Design review of the part built by this model. Coordinates are the model's own, in mm. Face numbers are marked on the shaded views. A direction names the side the tool comes from. Coordinates: 2 decimals unless noted, no trailing zeros. Write each loop counter-clockwise with the first axis right and the second up, starting at its lowest first coordinate (ties: lowest second). Pieces come first, ordered by that corner, then holes.
```python
from build123d import *

# Parameters (mm, degrees)
SKETCH1_W               = 54.356
SKETCH1_H               = 34.798
SKETCH1_R               = 1.250004527
SKETCH1_W_2             = 50.4000008
SKETCH1_H_2             = 5.2500022
BOSS_EXTRUDE1_DEPTH     = 1.999996
SKETCH2_W               = 54.356
SKETCH2_H               = 1.626997
BOSS_EXTRUDE2_DEPTH     = 4.1999916
SKETCH3_R               = 1.250004527
BOSS_EXTRUDE3_DEPTH     = 4.1999916
CUT_EXTRUDE1_DEPTH      = 33.88498208
CUT_EXTRUDE1_DEPTH_BACK = 33.88498208


with BuildPart() as part:
    # Sketch1 → Boss-Extrude1 (new body)
    with BuildSketch(Plane(origin=(0, 0, 0), x_dir=(1, 0, 0), z_dir=(0, 1, 0))):
        Rectangle(SKETCH1_W, SKETCH1_H)
        with Locations(Location((24.178011673, 3.099006966, 0), (0, 0, 270))):
            Circle(SKETCH1_R, mode=Mode.SUBTRACT)
        with Locations(Location((24.178011673, -3.099006966, 0), (0, 0, 90))):
            Circle(SKETCH1_R, mode=Mode.SUBTRACT)
        with Locations(Location((-24.178011673, -3.099006966, 0), (0, 0, 270))):
            Circle(SKETCH1_R, mode=Mode.SUBTRACT)
        with Locations(Location((-24.178011673, 3.099006966, 0), (0, 0, 90))):
            Circle(SKETCH1_R, mode=Mode.SUBTRACT)
        with Locations((-0.0219964, 11.7740049)):
            Rectangle(SKETCH1_W_2, SKETCH1_H_2, mode=Mode.SUBTRACT)
        with Locations((-0.0219964, -11.7740049)):
            Rectangle(SKETCH1_W_2, SKETCH1_H_2, mode=Mode.SUBTRACT)
    extrude(amount=BOSS_EXTRUDE1_DEPTH)

    # Sketch2 → Boss-Extrude2 (add)
    with BuildSketch(Plane(origin=(0, 1.999996, 0), x_dir=(1, 0, 0), z_dir=(0, 1, 0))):
        with Locations((0, 16.5855015)):
            Rectangle(SKETCH2_W, SKETCH2_H)
        with Locations((0, -16.5855015)):
            Rectangle(SKETCH2_W, SKETCH2_H)
    extrude(amount=BOSS_EXTRUDE2_DEPTH)

    # Sketch3 → Boss-Extrude3 (add)
    # profile 1 of 2: a face of its own
    with BuildSketch(Plane(origin=(0, 1.999996, 0), x_dir=(1, 0, 0), z_dir=(0, 1, 0))):
        Polygon((-27.207664346, 7.5999975), (-9.294212746, 7.5999975), (-10.799929046, 6.1000005), (-21.665998246, 6.1000005), (-21.665998246, -6.1000005), (-10.799929046, -6.1000005), (-9.294212746, -7.5999975), (-27.207664346, -7.5999975), align=None)
        with Locations(Location((-24.178011673, -3.099006966, 0), (0, 0, 270))):
            Circle(SKETCH3_R, mode=Mode.SUBTRACT)
        with Locations(Location((-24.178011673, 3.099006966, 0), (0, 0, 90))):
            Circle(SKETCH3_R, mode=Mode.SUBTRACT)
    # profile 2 of 2: a face of its own
    with BuildSketch(Plane(origin=(0, 1.999996, 0), x_dir=(1, 0, 0), z_dir=(0, 1, 0))):
        Polygon((27.207664346, -7.5999975), (9.294212746, -7.5999975), (10.799929046, -6.1000005), (21.665998246, -6.1000005), (21.665998246, 6.1000005), (10.799929046, 6.1000005), (9.294212746, 7.5999975), (27.207664346, 7.5999975), align=None)
        with Locations(Location((24.178011673, 3.099006966, 0), (0, 0, 90))):
            Circle(SKETCH3_R, mode=Mode.SUBTRACT)
        with Locations(Location((24.178011673, -3.099006966, 0), (0, 0, 90))):
            Circle(SKETCH3_R, mode=Mode.SUBTRACT)
    extrude(amount=BOSS_EXTRUDE3_DEPTH)

    # Sketch4 → Cut-Extrude1 (cut, two sides: drawn at the far end of the back side and taken through both)
    with BuildSketch(Plane.XZ.offset(-CUT_EXTRUDE1_DEPTH_BACK)):
        with BuildLine():
            ThreePointArc((-5.694081512, -3.1348976), (6.500011325, 0), (-5.694081512, 3.1348976))
            ThreePointArc((-5.694081512, 3.1348976), (-8.840003041, 0), (-5.694081512, -3.1348976))
        make_face()
        with BuildLine():
            ThreePointArc((-6.817717046, 5.7234709), (-12.015990113, 0), (-6.817717046, -5.7234709))
            Line((-6.817717046, -5.7234709), (-6.457037046, -6.1000005))
            Line((-6.457037046, -6.1000005), (-10.799929046, -6.1000005))
            Line((-10.799929046, -6.1000005), (-21.665998246, -6.1000005))
            Line((-21.665998246, -6.1000005), (-21.665998246, 6.1000005))
            Line((-21.665998246, 6.1000005), (-10.799929046, 6.1000005))
            Line((-10.799929046, 6.1000005), (-6.457037046, 6.1000005))
            Line((-6.457037046, 6.1000005), (-6.817717046, 5.7234709))
        make_face()
        with BuildLine():
            Line((6.457037046, 6.1000005), (6.817717046, 5.7234709))
            ThreePointArc((6.817717046, 5.7234709), (8.544974069, 0), (6.817717046, -5.7234709))
            Line((6.817717046, -5.7234709), (6.457037046, -6.1000005))
            Line((6.457037046, -6.1000005), (10.799929046, -6.1000005))
            Line((10.799929046, -6.1000005), (21.665998246, -6.1000005))
            Line((21.665998246, -6.1000005), (21.665998246, 6.1000005))
            Line((21.665998246, 6.1000005), (10.799929046, 6.1000005))
            Line((10.799929046, 6.1000005), (6.457037046, 6.1000005))
        make_face()
    extrude(amount=CUT_EXTRUDE1_DEPTH + CUT_EXTRUDE1_DEPTH_BACK, mode=Mode.SUBTRACT)


solid = part.part
```
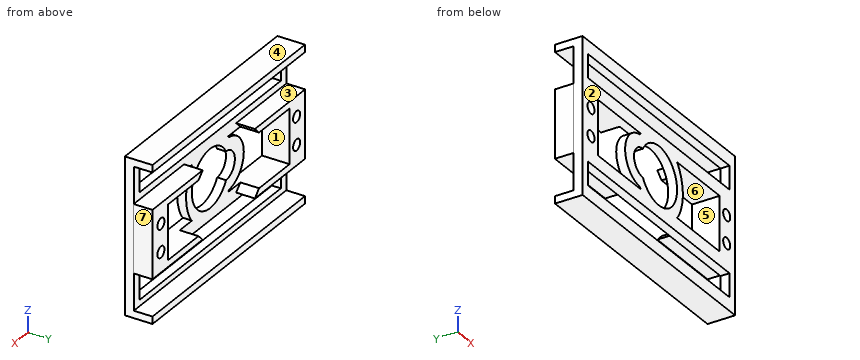
(1) Insertion check: pin 1 Ø6 at (x, z) = (-1.5, 10) entering from +Y; pin 2 Ø1 at (y, z) = (1, 12.5) entering from +X; pin 3 Ø1.6 at (y, z) = (1, -10.5) entering from -X. Each pin has a flat end and moves straight along its axis. Give the tip position at first contact, or say it passes through.
(2) Consider section A-A (z = -13). Give the boundary of the cut face in (x, y), plus the area to 3 significant figures.
(3) For the marked faces 1, 2 and 3, list the 3-axis set-ups (+Z, -Z, +X, -X, +Y, -Y) from which the entire face can be reached by the end or side of a thin tool; tool diameter is ignored.
(4) Mouldability with a two-part tool opening along X and no side actions: class the marked faces 4, 5, 6 and 7 as +X half, -X half, draft (parallel to the pull), parting line (faces both ways), or undercut.
(5) Consider section B-B (y = 5.5). Give the boundary of the cut face in (x, z).
(6) Consider section D-D (z = 0). State how many separate pieces and enclosed holes the cut face has, plus the area to 3 significant figures.
(7) Consider section C-C (x = 0). Give the boundary of the cut face in (y, z), plus the area to 3 significant figures.
(8) Wall thickness on line 1 (Z direction, x = 12.5, y = 0.5); line 2 (Z direction, x = -22, y = 4.25); line 3 (Z direction, x = -15, y = 4.5): over which ranges is each line inside the solid? List them lowest first.
Results:
1. pin 1: stops at y = 2
1. pin 2: stops at x = 27.18
1. pin 3: stops at x = -27.18
2. outline: (-27.18, 0) - (-25.22, 0) - (-25.22, 2) - (-27.18, 2) - close; (25.18, 0) - (27.18, 0) - (27.18, 2) - (25.18, 2) - close
2. area: 7.91 mm2
3. face 1: +Y, -Y
3. face 2: +Z, -Z, +X, -X, -Y
3. face 3: +X, -X, +Y
4. face 4: draft
4. face 5: undercut
4. face 6: undercut
4. face 7: +X half
5. outline: (-27.21, -7.6) - (-9.29, -7.6) - (-10.8, -6.1) - (-21.67, -6.1) - (-21.67, 6.1) - (-10.8, 6.1) - (-9.29, 7.6) - (-27.21, 7.6) - close; (-27.18, -17.4) - (27.18, -17.4) - (27.18, -15.77) - (-27.18, -15.77) - close; (-27.18, 15.77) - (27.18, 15.77) - (27.18, 17.4) - (-27.18, 17.4) - close; (9.29, -7.6) - (27.21, -7.6) - (27.21, 7.6) - (9.29, 7.6) - (10.8, 6.1) - (21.67, 6.1) - (21.67, -6.1) - (10.8, -6.1) - close; hole circle Ø2.5 at (-24.18, -3.1); hole circle Ø2.5 at (-24.18, 3.1); hole circle Ø2.5 at (24.18, -3.1); hole circle Ø2.5 at (24.18, 3.1)
6. separate pieces: 4
6. enclosed holes: 0
6. area: 79.0 mm2
7. outline: (0, -17.4) - (6.2, -17.4) - (6.2, -15.77) - (2, -15.77) - (2, -14.4) - (0, -14.4) - close; (0, -9.15) - (2, -9.15) - (2, -6.5) - (0, -6.5) - close; (0, 6.5) - (2, 6.5) - (2, 9.15) - (0, 9.15) - close; (0, 14.4) - (2, 14.4) - (2, 15.77) - (6.2, 15.77) - (6.2, 17.4) - (0, 17.4) - close
7. area: 36.3 mm2
8. line 1: z = -17.4 to -14.4, -9.15 to -6.1, 6.1 to 9.15, 14.4 to 17.4
8. line 2: z = -17.4 to -15.77, -7.6 to 7.6, 15.77 to 17.4
8. line 3: z = -17.4 to -15.77, -7.6 to -6.1, 6.1 to 7.6, 15.77 to 17.4
